from build123d import *

# Parameters (mm, degrees)
BOX004_W     = 20
BOX004_H     = 30
BOX004_DEPTH = 10
BOX003_W     = 20
BOX003_H     = 30
BOX003_DEPTH = 10
BOX002_W     = 22
BOX002_H     = 22
BOX002_DEPTH = 10
BOX001_W     = 22
BOX001_H     = 22
BOX001_DEPTH = 10
BOX_W        = 390
BOX_H        = 260
BOX_DEPTH    = 4


with BuildPart() as corte_rail_der:
    # Box004 → Box004 (new body)
    with BuildSketch(Plane(origin=(245, 230, -3), x_dir=(1, 0, 0), z_dir=(0, 0, 1))):
        with Locations((10, 15)):
            Rectangle(BOX004_W, BOX004_H)
    extrude(amount=BOX004_DEPTH)


with BuildPart() as obj1:
    # Box003 → Box003 (new body)
    with BuildSketch(Plane(origin=(125, 230, -3), x_dir=(1, 0, 0), z_dir=(0, 0, 1))):
        with Locations((10, 15)):
            Rectangle(BOX003_W, BOX003_H)
    extrude(amount=BOX003_DEPTH)


with BuildPart() as corte_der:
    # Box002 → Box002 (new body)
    with BuildSketch(Plane(origin=(368, 0, -3), x_dir=(1, 0, 0), z_dir=(0, 0, 1))):
        with Locations((11, 11)):
            Rectangle(BOX002_W, BOX002_H)
    extrude(amount=BOX002_DEPTH)


with BuildPart() as obj2:
    # Box001 → Box001 (new body)
    with BuildSketch(Plane.XY.offset(-3)):
        with Locations((11, 11)):
            Rectangle(BOX001_W, BOX001_H)
    extrude(amount=BOX001_DEPTH)


with BuildPart() as obj3:
    # Box → Box (new body)
    with BuildSketch(Plane.XY):
        with Locations((195, 130)):
            Rectangle(BOX_W, BOX_H)
    extrude(amount=BOX_DEPTH)

    # Cut: cut obj2
    add(obj2.part, mode=Mode.SUBTRACT)

    # Cut001: cut corte_der
    add(corte_der.part, mode=Mode.SUBTRACT)

    # Cut002: cut obj1
    add(obj1.part, mode=Mode.SUBTRACT)

    # Cut003: cut corte_rail_der
    add(corte_rail_der.part, mode=Mode.SUBTRACT)


solid = obj3.part
Read the model definition and answer for the solid it produces. Units are mm, in the model's axes. Give positions to 0.01 mm unless a question says otherwise; leave off trailing zeros. Loops run counter-clockwise (first coordinate to the right, second up) from the corner with the lowest first, then second, coordinate; pieces in that order, holes last. Notation, with made-up numbers: (17.5, -35.5) - (76.5, -35.5) arc R23 ccw to (76.5, -23.5) - close; hole circle Ø5 at (-2.5, 54). An arc over 180 degrees is marked (long way). Answer as CSV lines item,"result". Start each with the question number.
1) Each of these flat-tipped pins is pushed along its axis until it touches: pin 1 Ø1.2 at (y, z) = (7, 1) entering from -X; pin 2 Ø1.2 at (y, z) = (7.5, 2.5) entering from +X. Where does it stop, or does it pass through?
2) Find section B-B (x = 141). Write down the section's boundary in (y, z), then the cut area to 3 significant figures.
3) Find section A-A (z = 2.8). Write down the section's boundary in (x, y), then the cut area to 3 significant figures.
4) Straight lines are drawn through the part: L1, parallel to X at y = 233, z = 3.8; L2, parallel to Y at x = 371, z = 2.15; L3, parallel to Y at x = 138, z = 1.25. For each, find the intervals that lie inside material, in ascending order. Write a range as from..to.
Findings below:
1,pin 1,"x = 22"
1,pin 2,"x = 368"
2,outline,"(0, 0) - (230, 0) - (230, 4) - (0, 4) - close"
2,area,"920 mm^2"
3,outline,"(0, 22) - (22, 22) - (22, 0) - (368, 0) - (368, 22) - (390, 22) - (390, 260) - (265, 260) - (265, 230) - (245, 230) - (245, 260) - (145, 260) - (145, 230) - (125, 230) - (125, 260) - (0, 260) - close"
3,area,"99,200 mm^2"
4,L1,"0..125, 145..245, 265..390"
4,L2,"22..260"
4,L3,"0..230"
